For this review, take the finished solid that the model builds, in its own axes (mm). Face numbers are marked on the shaded views. A direction names the side the tool comes from. Round coordinates to 2 decimals unless told otherwise and drop trailing zeros. Write each loop counter-clockwise with the first axis right and the second up, starting at its lowest first coordinate (ties: lowest second). Pieces come first, ordered by that corner, then holes. Notation, with made-up numbers: (75, 46) -> (106, 46) arc R24 cw to (106, 75) -> close; hole circle Ø7 at (51.5, -15.75). An arc over 180 degrees is marked (long way). Answer in a Markdown table with one row per item.
from build123d import *

# Parameters (mm, degrees)
F0_W     = 2150
F0_H     = 600
F1_DEPTH = 50
F2_W     = 2090
F2_H     = 500
F3_DEPTH = 900
F4_W     = 640
F4_H     = 120
F4_W_2   = 650
F4_W_3   = 312.5
F4_H_2   = 560
F4_W_4   = 317.5
F4_W_5   = 322.5
F5_DEPTH = 30
F6_W     = 2030
F6_H     = 900
F7_DEPTH = 200


with BuildPart() as f1:
    # F0 (on Top) → F1 (new body)
    with BuildSketch(Plane.XY):
        Rectangle(F0_W, F0_H)
    extrude(amount=F1_DEPTH)

    # F2 (on Top) → F3 (join)
    with BuildSketch(Plane.XY):
        Rectangle(F2_W, F2_H)
    extrude(amount=-F3_DEPTH)

    # F4 (on face) → F5 (join)
    with BuildSketch(Plane.XZ.offset(250)):
        with Locations((-695, -110)):
            Rectangle(F4_W, F4_H)
        with Locations((0, -110)):
            Rectangle(F4_W_2, F4_H)
        with Locations((695, -110)):
            Rectangle(F4_W, F4_H)
        with Locations((-858.75, -470)):
            Rectangle(F4_W_3, F4_H_2)
        with Locations((-533.75, -470)):
            Rectangle(F4_W_4, F4_H_2)
        with Locations((-166.25, -470)):
            Rectangle(F4_W_4, F4_H_2)
        with Locations((163.75, -470)):
            Rectangle(F4_W_5, F4_H_2)
        with Locations((531.25, -470)):
            Rectangle(F4_W_3, F4_H_2)
        with Locations((856.25, -470)):
            Rectangle(F4_W_4, F4_H_2)
    extrude(amount=F5_DEPTH)

    # F6 (on face) → F7 (cut)
    with BuildSketch(Plane(origin=(0, 250, 0), x_dir=(-1, 0, 0), z_dir=(0, 1, 0))):
        with Locations((0, -450)):
            Rectangle(F6_W, F6_H)
    extrude(amount=-F7_DEPTH, mode=Mode.SUBTRACT)


solid = f1.part
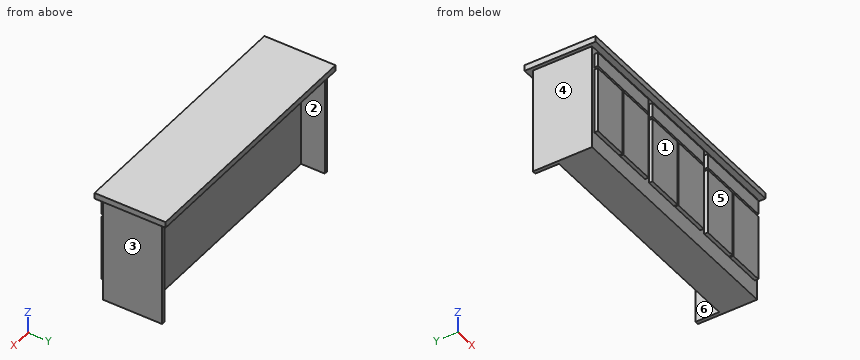
1) Mouldability with a two-part tool opening along X and no side actions: class the marked faces 1, 2 and 3 as pulls with the +X half, pulls with the -X half, needs draft (parallel to the pull), parting line crosses it, or undercut.
Solved:
| item | result |
|---|---|
| face 1 | needs draft |
| face 2 | undercut |
| face 3 | pulls with the +X half |
2) For line 1 (X direction, y = 230, z = -212.5); line 2 (Z direction, x = 919.5, y = 57); line 3 (X direction, y = -90, z = -710), list the stretches that pass through material, from the lowest coordinate up. Write a range as [from, to].
Solved:
| item | result |
|---|---|
| line 1 | [-1045, -1015], [1015, 1045] |
| line 2 | [0, 50] |
| line 3 | [-1045, 1045] |
3) For the marked faces 4, 5 and 6, list the 3-axis set-ups (+Z, -Z, +X, -X, +Y, -Y) from which the entire face can be reached by the end or side of a thin tool; tool diameter is ignored.
Solved:
| item | result |
|---|---|
| face 4 | -Z, -X, +Y, -Y |
| face 5 | -Z, +X, -X, -Y |
| face 6 | -Z, +Y |
4) Clearance check with flat-ended pins moving along their axes: pin 1 Ø24 at (x, y) = (-882.5, -267) entering from -Z; pin 2 Ø8 at (x, z) = (675.5, -172.5) entering from +Y; pin 3 Ø9 at (y, z) = (-270, -505.5) entering from -X. State where each tip first meets the part, or that it passes through.
Solved:
| item | result |
|---|---|
| pin 1 | z = -750 |
| pin 2 | y = 50 |
| pin 3 | x = -1015 |
5) Consider section C-C on y = -130.5. State the section outline as (x, z) points, then the cut area to 3 significant figures.
Solved:
| item | result |
|---|---|
| outline | (-1075, 0) -> (-1045, 0) -> (-1045, -900) -> (1045, -900) -> (1045, 0) -> (1075, 0) -> (1075, 50) -> (-1075, 50) -> close |
| area | 1,990,000 mm² |
6) Consider section B-B on x = 608.5. State the section outline as (y, z) points, then the cut area to 3 significant figures.
Solved:
| item | result |
|---|---|
| outline | (-300, 0) -> (-250, 0) -> (-250, -50) -> (-280, -50) -> (-280, -170) -> (-250, -170) -> (-250, -190) -> (-280, -190) -> (-280, -750) -> (-250, -750) -> (-250, -900) -> (50, -900) -> (50, 0) -> (300, 0) -> (300, 50) -> (-300, 50) -> close |
| area | 320,000 mm² |
7) Consider section D-D on z = -115. State the section outline as (x, y) points, then the cut area to 3 significant figures.
Solved:
| item | result |
|---|---|
| outline | (-1045, -250) -> (-1015, -250) -> (-1015, -280) -> (-375, -280) -> (-375, -250) -> (-325, -250) -> (-325, -280) -> (325, -280) -> (325, -250) -> (375, -250) -> (375, -280) -> (1015, -280) -> (1015, -250) -> (1045, -250) -> (1045, 250) -> (1015, 250) -> (1015, 50) -> (-1015, 50) -> (-1015, 250) -> (-1045, 250) -> close |
| area | 697,000 mm² |
